Here's the drawing with two shaded views (mm, measured from the low corner). I have some questions. A direction names the side the tool comes from. Coordinates: 2 decimals unless noted, no trailing zeros. Write each loop counter-clockwise with the first axis right and the second up, starting at its lowest first coordinate (ties: lowest second). Pieces come first, ordered by that corner, then holes. Notation, with made-up numbers: (66.25, 56) -> (74.25, 56) arc R22 cw to (74.25, 74) -> close; hole circle Ø10 at (31, 58.25). An arc over 180 degrees is marked (long way). Put each result on its own line as item: value.
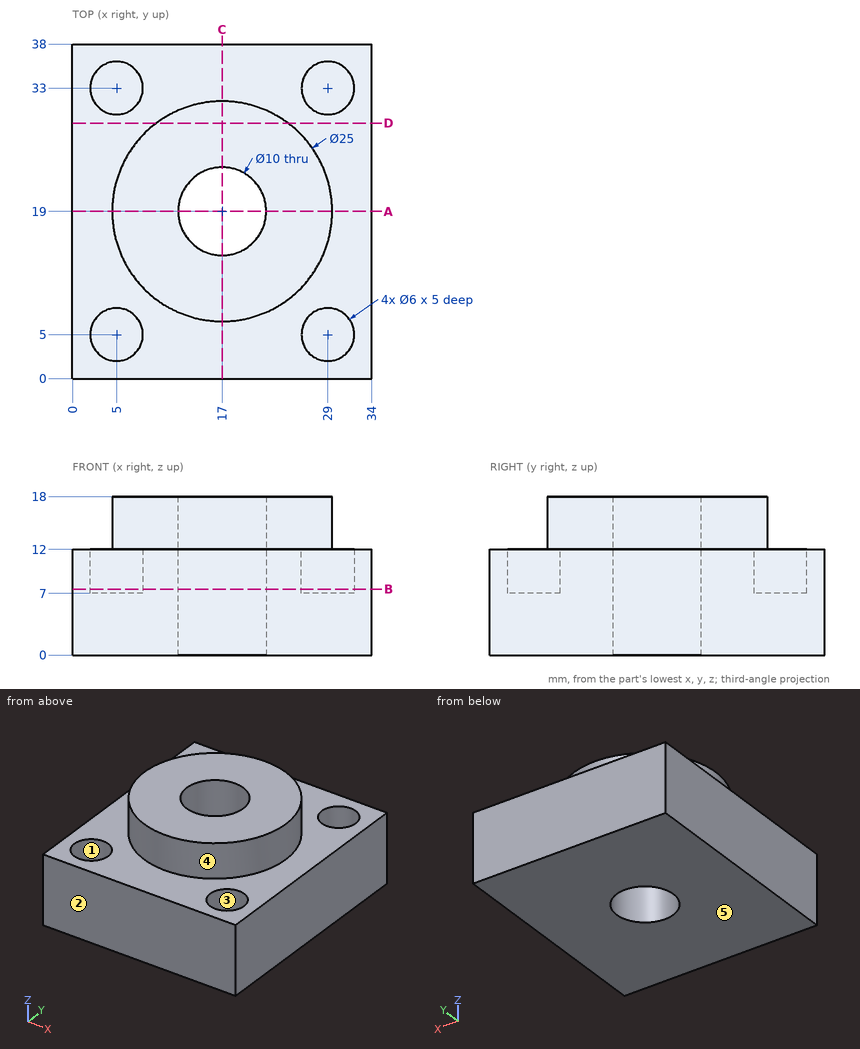
Item 1: Which directions (+Z, -Z, +X, -X, +Y, -Y) give clear straight access to the entire face, cutting with the end or side of a thin tool? Please do the marked faces 1 and 2.
Output:
face 1: +Z
face 2: +Z, -Z, +X, -X, -Y
Item 2: If we mould it in two halves opening along Y, with no side actions, what happens to the marked faces 3, 4 and 5? For each: released by +Y, released by -Y, zero draft, split by the parting line, or undercut.
Output:
face 3: undercut
face 4: split by the parting line
face 5: zero draft
Item 3: Imagine slicing it at C-C on x = 17. Write out the boundary of the cut face in (y, z), then the cut area to 3 significant figures.
Output:
outline: (0, 0) -> (14, 0) -> (14, 18) -> (6.5, 18) -> (6.5, 12) -> (0, 12) -> close; (24, 0) -> (38, 0) -> (38, 12) -> (31.5, 12) -> (31.5, 18) -> (24, 18) -> close
area: 426 mm²
Item 4: Imagine slicing it at D-D on y = 29. Write out the boundary of the cut face in (x, z).
Output:
outline: (0, 0) -> (34, 0) -> (34, 12) -> (24.5, 12) -> (24.5, 18) -> (9.5, 18) -> (9.5, 12) -> (0, 12) -> close
Item 5: Please list where these lines run through material, in increasing order: line 1 along Y through (x, z) = (29, 10.1); line 2 along Y through (x, z) = (17, 14); line 3 along Y through (x, z) = (28, 10). Write a range as from..to.
Output:
line 1: y = 0..2, 8..30, 36..38
line 2: y = 6.5..14, 24..31.5
line 3: y = 0..2.17, 7.83..30.17, 35.83..38
Item 6: For P1, Ø6.5, axis at x = 30.5, y = 4, coming from the +Z side; P2, Ø5.5, axis at x = 29, y = 33, coming from the +Z side; P3, Ø1.5, axis at x = 25.5, z = 13, coming from the +Y side, each with a flat end and sliding along its axis, tell me the tip position at first contact or that it passes through.
Output:
P1: stops at z = 12
P2: stops at z = 7
P3: stops at y = 28.81
Item 7: Imagine slicing it at A-A on y = 19. Write out the boundary of the cut face in (x, z), then the cut area to 3 significant figures.
Output:
outline: (0, 0) -> (12, 0) -> (12, 18) -> (4.5, 18) -> (4.5, 12) -> (0, 12) -> close; (22, 0) -> (34, 0) -> (34, 12) -> (29.5, 12) -> (29.5, 18) -> (22, 18) -> close
area: 378 mm²
Item 8: Imagine slicing it at B-B on z = 7.5. Write out the boundary of the cut face in (x, y).
Output:
outline: (0, 0) -> (34, 0) -> (34, 38) -> (0, 38) -> close; hole circle Ø6 at (5, 5); hole circle Ø6 at (5, 33); hole circle Ø10 at (17, 19); hole circle Ø6 at (29, 5); hole circle Ø6 at (29, 33)
